Geometry: final body of the model. Coordinates: model frame, mm. A direction names the side the tool comes from. Coordinates: 2 decimals unless noted, no trailing zeros. Order: outer loops, then holes, each group sorted by start corner. A loop starts at its lowest first (then second) coordinate and runs counter-clockwise, first axis right, second up. Notation, with made-up numbers: M 52,-1 L 110,-1 A27 cw 110,27 Z; hole C 56,15 d4. An arc over 180 degrees is marked long. Use CSV: the item, a comma, the result in double quotes. Start each with the question number.
Q1. Access query for faces 3 (the face through (0, -2, -12.7)), 4 (the face through (1, -2, 0)). Directions: +Z, -Z, +X, -X, +Y, -Y. A direction counts if a zero-diameter tool reaches every point of the face in a straight line with its end or side. Return the directions, or none.
Q2. First-contact query: P1, Ø1.5, axis at x = 0.5, y = -1, coming from the -Z side. Flat tip, straight axial feed; report the tip coordinate or a pass-through.
Q3. Ray query, probe 1 along Y at (x, z) = (0, -17) (3 decimals); probe 2 along Z at (x, y) = (-1.25, 1.75). Return the intervals inside material, ascending.
Q4. Mould query, pull axis X, two halves, no side actions, for faces 1 (the face through (-0.25, -1.87, -6.44)), 2 (the face through (-1.4, -2.1, -33.78)). Classes: +X half, -X half, draft (parallel to the pull), parting line (faces both ways), or undercut.
Q5. Section query A-A, the plane z = -29. Output: boundary loops of the cut face in (x, y) (3 decimals), and give its area (3 significant figures).
from build123d import *

# Parameters (mm, degrees)
SKETCH1_R           = 3.175
SKETCH1_R_2         = 2.286
BOSS_EXTRUDE1_DEPTH = 29.7165
SKETCH2_R           = 3.175
SKETCH2_R_2         = 2.286
BOSS_EXTRUDE2_DEPTH = 4.064
SKETCH3_R           = 2.762
SKETCH3_R_2         = 2
EXTRUDE_THIN1_DEPTH = 12.7
EXTRUDE_THIN1_TAPER = -1


with BuildPart() as part:
    # Sketch1 → Boss-Extrude1 (new body)
    with BuildSketch(Plane.XY):
        Circle(SKETCH1_R)
        Circle(SKETCH1_R_2, mode=Mode.SUBTRACT)
    extrude(amount=-BOSS_EXTRUDE1_DEPTH)

    # Sketch2 → Boss-Extrude2 (add)
    with BuildSketch(Plane(origin=(0, 0, -29.7165), x_dir=(-1, 0, 0), z_dir=(0, 0, -1))):
        Circle(SKETCH2_R)
        Circle(SKETCH2_R_2, mode=Mode.SUBTRACT)
    extrude(amount=BOSS_EXTRUDE2_DEPTH)

    # Sketch3 → Extrude-Thin1 (add)
    with BuildSketch(Plane.XY):
        Circle(SKETCH3_R)
        Circle(SKETCH3_R_2, mode=Mode.SUBTRACT)
    extrude(amount=-EXTRUDE_THIN1_DEPTH, taper=EXTRUDE_THIN1_TAPER)


solid = part.part
Responses:
1,face 3,"-Z"
1,face 4,"+Z, +X, -X, +Y, -Y"
2,P1,"stops at z = -12.7"
3,probe 1,"y = -3.175 to -2.286, 2.286 to 3.175"
3,probe 2,"z = -12.7 to 0"
4,face 1,"undercut"
4,face 2,"draft"
5,outline,"C 0,0 d6.35; hole C 0,0 d4.572"
5,area,"15.3 mm²"
